```python
from build123d import *

# Parameters (mm, degrees)
CUT_EXTRUDE1_DEPTH      = 8.5
CUT_EXTRUDE1_DEPTH_BACK = 8.5
SKETCH3_R               = 3.75
CUT_EXTRUDE2_DEPTH      = 11.5
CHAMFER1_SIZE           = 3
CHAMFER1_SIZE2          = 5
CHAMFER1_PART_2_SIZE    = 3
CHAMFER1_PART_2_SIZE2   = 5
SKETCH4_R               = 3
CUT_EXTRUDE3_DEPTH      = 27.5
SKETCH5_R               = 1.5
CUT_EXTRUDE4_DEPTH      = 8.5000001
CUT_EXTRUDE4_DEPTH_BACK = 8.5000001


with BuildPart() as part:
    # Sketch1 → Revolve1 (revolve)
    with BuildSketch(Plane(origin=(0, 0, 0), x_dir=(0, 0, -1), z_dir=(1, 0, 0))):
        Polygon((0, 4), (36, 4), (36, 6), (41, 6), (41, 7.5), (54.5, 7.5), (54.5, 0), (0, 0), align=None)
    revolve(axis=Axis((0, 0, 0), (0, 0, -1)))

    # Sketch2 → Cut-Extrude1 (cut, two sides)
    with BuildSketch(Plane(origin=(0, 0, 0), x_dir=(0, 0, -1), z_dir=(1, 0, 0))) as cut_extrude1_sk:
        with BuildLine():
            Line((54.5, -1.5), (45, -1.5))
            ThreePointArc((45, -1.5), (43.5, 0), (45, 1.5))
            Line((45, 1.5), (54.5, 1.5))
            ThreePointArc((54.5, 1.5), (56, 0), (54.5, -1.5))
        make_face()
    extrude(amount=CUT_EXTRUDE1_DEPTH, mode=Mode.SUBTRACT)
    extrude(cut_extrude1_sk.sketch, amount=-CUT_EXTRUDE1_DEPTH_BACK, mode=Mode.SUBTRACT)

    # Sketch3 → Cut-Extrude2 (cut)
    with BuildSketch(Plane(origin=(0, 0, -54.5), x_dir=(-1, 0, 0), z_dir=(0, 0, -1))):
        Circle(SKETCH3_R)
    extrude(amount=-CUT_EXTRUDE2_DEPTH, mode=Mode.SUBTRACT)

    # Chamfer1
    chamfer1_edges = [part.edges().sort_by_distance(p)[0] for p in [
        (0, -3.75, -54.5),
    ]]
    chamfer1_side = [part.faces().sort_by_distance(p)[0] for p in [
        (0, -4.328722243, -54.5),
    ]]
    chamfer(chamfer1_edges, length=CHAMFER1_SIZE, length2=CHAMFER1_SIZE2, reference=chamfer1_side[0])

    # Chamfer1 part 2
    chamfer1_part_2_edges = [part.edges().sort_by_distance(p)[0] for p in [
        (0, 3.75, -54.5),
    ]]
    chamfer1_part_2_side = [part.faces().sort_by_distance(p)[0] for p in [
        (0, 4.328722243, -54.5),
    ]]
    chamfer(chamfer1_part_2_edges, length=CHAMFER1_PART_2_SIZE, length2=CHAMFER1_PART_2_SIZE2, reference=chamfer1_part_2_side[0])

    # Sketch4 → Cut-Extrude3 (cut)
    with BuildSketch(Plane.XY):
        Circle(SKETCH4_R)
    extrude(amount=-CUT_EXTRUDE3_DEPTH, mode=Mode.SUBTRACT)

    # Sketch5 → Cut-Extrude4 (cut, two sides)
    with BuildSketch(Plane(origin=(0, 0, 0), x_dir=(0, -1, 0), z_dir=(1, 0, 0))) as cut_extrude4_sk:
        with Locations((0, 19.5)):
            Circle(SKETCH5_R)
    extrude(amount=CUT_EXTRUDE4_DEPTH, mode=Mode.SUBTRACT)
    extrude(cut_extrude4_sk.sketch, amount=-CUT_EXTRUDE4_DEPTH_BACK, mode=Mode.SUBTRACT)


solid = part.part
```
Geometry check sheet. Reference: the model listing, model coordinates, mm. A direction names the side the tool comes from. Give positions to 0.01 mm unless a question says otherwise; leave off trailing zeros. Write each loop counter-clockwise with the first axis right and the second up, starting at its lowest first coordinate (ties: lowest second). Pieces come first, ordered by that corner, then holes.
1) Access from +Z, -Z, +X, -X, +Y, -Y to the whole of each face (thin tool, end or side, straight path). Record for faces 4 (the flat face through (-6, -1.5, -49)), 5 (the flat face through (0, 0, -43)), 6 (the cylindrical face through (3.29, -1.386, -18.925)), 7 (the cylindrical face through (-3, 0, -14)).
2) Release check for a two-part mould opening along Z. For faces 1 (the cylindrical face through (-3.29, -1.386, -18.925)), 2 (the conical face through (-0.092, 4.895, -51.409)), 3 (the flat face through (6, -2, -41)) record: pulls with the +Z half, pulls with the -Z half, needs draft (parallel to the pull), parting line crosses it, or undercut.
3) Material ranges on L1, parallel to Z at x = -3.4, y = 0; L2, parallel to Y at x = 0, z = -45; L3, parallel to Z at x = -2.85, y = 0, recorded low to high.
4) Section check A-A, the plane z = -46. Record the boundary of the cut face in (x, y).
5) Section check B-B, the plane y = -0.5. Record the boundary of the cut face in (x, z).
6) Section check C-C, the plane x = 0. Record the boundary of the cut face in (y, z), and give its area (3 significant figures).
7) Section check D-D, the plane z = -12. Record the boundary of the cut face in (x, y).
8) Gauge pin test, flat ends, axial feed: pin 1 (5 mm diameter, centred on y = -1.5, z = -29.5, fed in from -X); pin 2 (1.8 mm diameter, centred on y = 0, z = -19.5, fed in from +X); pin 3 (4 mm diameter, centred on x = 1.5, y = 1.5, fed in from -Z); pin 4 (3 mm diameter, centred on x = 5, z = -51, fed in from -Y). Record the tip position at first contact, or that the pin passes through.
Computed:
1. face 4: -Z, +X, -X
1. face 5: -Z
1. face 6: +X, -X
1. face 7: +Z
2. face 1: undercut
2. face 2: pulls with the -Z half
2. face 3: pulls with the +Z half
3. L1: z = -43 to -21, -18 to 0
3. L2: y = -7.5 to -3.75, 3.75 to 7.5
3. L3: z = -43 to -27.5
4. outline: (-7.35, -1.5) arc R7.5 ccw to (7.35, -1.5) - (3.44, -1.5) arc R3.75 cw to (-3.44, -1.5) - close; (-7.35, 1.5) - (-3.44, 1.5) arc R3.75 cw to (3.44, 1.5) - (7.35, 1.5) arc R7.5 ccw to start
5. outline: (-7.48, -43.59) - (-3.72, -43.59) - (-3.72, -43) - (3.72, -43) - (3.72, -43.59) - (7.48, -43.59) - (7.48, -41) - (5.98, -41) - (5.98, -36) - (3.97, -36) - (3.97, -20.91) - (2.96, -20.91) - (2.96, -27.5) - (-2.96, -27.5) - (-2.96, -20.91) - (-3.97, -20.91) - (-3.97, -36) - (-5.98, -36) - (-5.98, -41) - (-7.48, -41) - close; (-3.97, -18.09) - (-2.96, -18.09) - (-2.96, 0) - (-3.97, 0) - close; (2.96, -18.09) - (3.97, -18.09) - (3.97, 0) - (2.96, 0) - close
6. outline: (-7.5, -54.5) - (-6.75, -54.5) - (-3.75, -49.5) - (-3.75, -43) - (3.75, -43) - (3.75, -49.5) - (6.75, -54.5) - (7.5, -54.5) - (7.5, -41) - (6, -41) - (6, -36) - (4, -36) - (4, 0) - (3, 0) - (3, -27.5) - (-3, -27.5) - (-3, 0) - (-4, 0) - (-4, -36) - (-6, -36) - (-6, -41) - (-7.5, -41) - close
6. area: 284 mm2
7. outline: circle Ø8 at (0, 0); hole circle Ø6 at (0, 0)
8. pin 1: stops at x = -4
8. pin 2: passes through
8. pin 3: stops at z = -50.12
8. pin 4: stops at y = -6.63
